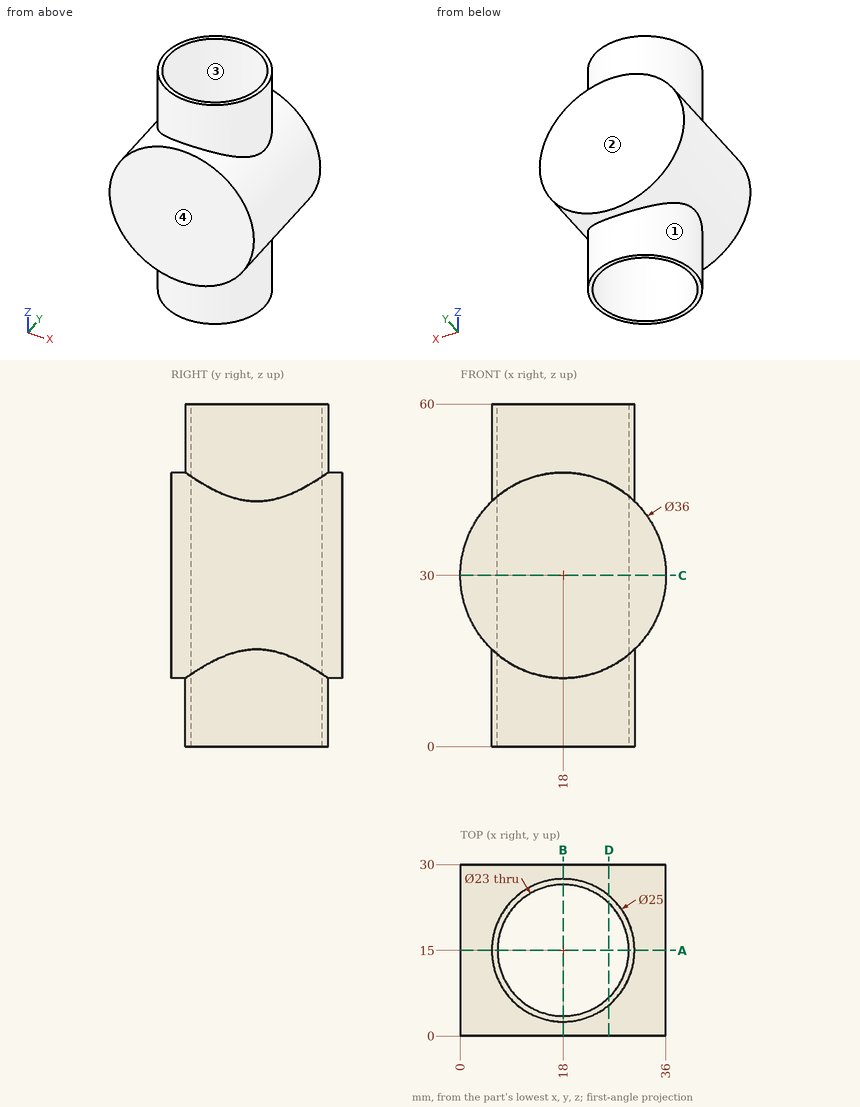
Can you work these out from the drawing? Everything is in mm from the part's minimum corner. Round coordinates to 2 decimals unless told otherwise and drop trailing zeros. Order: outer loops, then holes, each group sorted by start corner. A loop starts at its lowest first (then second) coordinate and runs counter-clockwise, first axis right, second up.
(1) We'd pull the mould along Y, two halves only. Please class the marked faces 1, 2, 3 and 4: +Y half, -Y half, draft (parallel to the pull), parting line (faces both ways), or undercut.
Results are:
face 1: parting line
face 2: +Y half
face 3: undercut
face 4: -Y half
(2) If we section it at D-D (x = 26): Please give me the cut outline in (y, z).
Results are:
outline: (0, 13.88) - (5.4, 13.88) - (5.4, 0) - (6.74, 0) - (6.74, 60) - (5.4, 60) - (5.4, 46.12) - (0, 46.12) - close; (23.26, 0) - (24.6, 0) - (24.6, 13.88) - (30, 13.88) - (30, 46.12) - (24.6, 46.12) - (24.6, 60) - (23.26, 60) - close
(3) I'm going to push flat-ended pins straight in: pin 1 (1.5 mm diameter, centred on y = 17, z = 48.5, fed in from +X); pin 2 (5 mm diameter, centred on x = 11.5, z = 52, fed in from +Y); pin 3 (10 mm diameter, centred on y = 22, z = 37.5, fed in from +X). Where does each tip first touch, or does it pass through?
Results are:
pin 1: stops at x = 30.44
pin 2: stops at y = 26.84
pin 3: stops at x = 35.83
(4) If we section it at C-C (z = 30): Please give me the cut outline in (x, y), plus the area to 3 significant figures.
Results are:
outline: (0, 0) - (36, 0) - (36, 30) - (0, 30) - close; hole circle Ø23 at (18, 15)
area: 665 mm2
(5) If we section it at A-A (y = 15): Please give me the cut outline in (x, z).
Results are:
outline: (5.5, 0) - (6.5, 0) - (6.5, 60) - (5.5, 60) - (5.5, 42.95) arc R18 ccw to (5.5, 17.05) - close; (29.5, 0) - (30.5, 0) - (30.5, 17.05) arc R18 ccw to (30.5, 42.95) - (30.5, 60) - (29.5, 60) - close
(6) If we section it at B-B (x = 18): Please give me the cut outline in (y, z), plus the area to 3 significant figures.
Results are:
outline: (0, 12) - (2.5, 12) - (2.5, 0) - (3.5, 0) - (3.5, 60) - (2.5, 60) - (2.5, 48) - (0, 48) - close; (26.5, 0) - (27.5, 0) - (27.5, 12) - (30, 12) - (30, 48) - (27.5, 48) - (27.5, 60) - (26.5, 60) - close
area: 300 mm2
(7) If I drill on L1, parallel to Y at x = 18, z = 15; L2, parallel to X at y = 22.5, z = 20.5; L3, parallel to X at y = 23, z = 14, over which ranges is the centre line in solid material (lowest first)?
Results are:
L1: y = 0 to 3.5, 26.5 to 30
L2: x = 2.71 to 9.28, 26.72 to 33.29
L3: x = 8.4 to 9.74, 26.26 to 27.6
